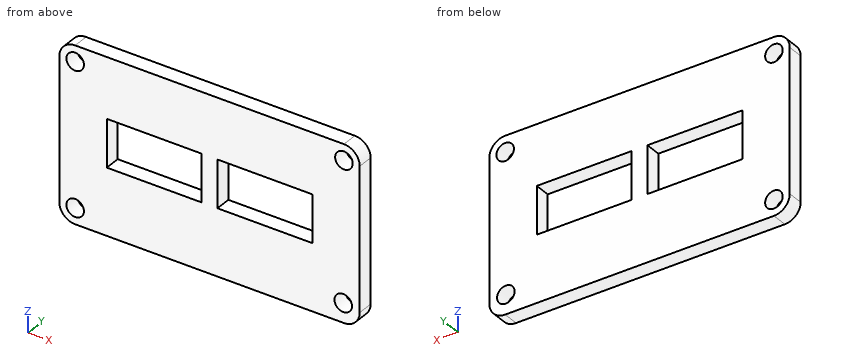
```python
from build123d import *

# Parameters (mm, degrees)
SKETCH1_W                   = 48.26
SKETCH1_H                   = 27.94
BOSS_EXTRUDE1_DEPTH         = 2.54
SKETCH2_W                   = 15.24
SKETCH2_H                   = 7.62
CUT_EXTRUDE1_DEPTH          = 15.494
FILLET1_R                   = 2.54
F_34_0_111_DIAMETER_HOLE1_D = 2.8194


with BuildPart() as part:
    # Sketch1 → Boss-Extrude1 (new body)
    with BuildSketch(Plane(origin=(0, 0, 0), x_dir=(1, 0, 0), z_dir=(0, 1, 0))):
        Rectangle(SKETCH1_W, SKETCH1_H)
    extrude(amount=BOSS_EXTRUDE1_DEPTH)

    # Sketch2 → Cut-Extrude1 (cut)
    with BuildSketch(Plane(origin=(0, 2.54, 0), x_dir=(1, 0, 0), z_dir=(0, 1, 0))):
        with Locations((-8.89, -0.508)):
            Rectangle(SKETCH2_W, SKETCH2_H)
        with Locations((8.89, -0.508)):
            Rectangle(SKETCH2_W, SKETCH2_H)
    extrude(amount=-CUT_EXTRUDE1_DEPTH, mode=Mode.SUBTRACT)

    # Fillet1
    fillet1_edges = [part.edges().sort_by_distance(p)[0] for p in [
        (-24.13, 1.27, 13.97),
        (-24.13, 1.27, -13.97),
        (24.13, 1.27, -13.97),
        (24.13, 1.27, 13.97),
    ]]
    fillet(fillet1_edges, radius=FILLET1_R)

    # #34 (0.111) Diameter Hole1 (through all)
    with Locations(Plane(origin=(0, 2.54, 0), x_dir=(1, 0, 0), z_dir=(0, 1, 0))):
        with Locations((21.483576639, 10.878336476), (21.59, -11.43), (-21.59, -11.43), (-21.59, 11.43)):
            Hole(F_34_0_111_DIAMETER_HOLE1_D / 2)


solid = part.part
```
Check sheet for the modelled part. Datum: model origin and axes. Units: mm. Give positions to 0.01 mm unless a question says otherwise; leave off trailing zeros. Loops run counter-clockwise (first coordinate to the right, second up) from the corner with the lowest first, then second, coordinate; pieces in that order, holes last. Notation, with made-up numbers: (-0.75, 30.5) - (6.25, 30.5) arc R26 ccw to (6.25, 48.5) - close; hole circle Ø2 at (72.25, 77.25). An arc over 180 degrees is marked (long way). One line per question, with ' | ' between items. Start each with the question number.
1. Material ranges on line 1 along X through (y, z) = (1.05, 2); line 2 along Z through (x, y) = (-21.59, 1.7); line 3 along Z through (x, y) = (-2, 0.9), recorded low to high. Write a range as [from, to].
2. Cross-section at B-B, the plane x = -6.5. Enter the section's corners in (y, z).
3. Gauge pin test, flat end, axial feed: pin 1 Ø2.5 at (x, z) = (-21.59, -11.43) entering from -Y. Record the tip position at first contact, or that the pin passes through.
4. Cross-section at C-C, the plane y = 1.85. Enter the section's corners in (x, z).
5. Cross-section at A-A, the plane z = 2.5. Enter the section's corners in (x, y).
Check result:
1) line 1: x = [-24.13, -16.51], [-1.27, 1.27], [16.51, 24.13] | line 2: z = [-13.97, -12.84], [-10.02, 10.02], [12.84, 13.97] | line 3: z = [-13.97, -3.3], [4.32, 13.97]
2) outline: (0, -13.97) - (2.54, -13.97) - (2.54, -3.3) - (0, -3.3) - close; (0, 4.32) - (2.54, 4.32) - (2.54, 13.97) - (0, 13.97) - close
3) pin 1: passes through
4) outline: (-24.13, -11.43) arc R2.54 ccw to (-21.59, -13.97) - (21.59, -13.97) arc R2.54 ccw to (24.13, -11.43) - (24.13, 11.43) arc R2.54 ccw to (21.59, 13.97) - (-21.59, 13.97) arc R2.54 ccw to (-24.13, 11.43) - close; hole circle Ø2.82 at (-21.59, -11.43); hole circle Ø2.82 at (-21.59, 11.43); hole (-16.51, -3.3) - (-1.27, -3.3) - (-1.27, 4.32) - (-16.51, 4.32) - close; hole (1.27, -3.3) - (16.51, -3.3) - (16.51, 4.32) - (1.27, 4.32) - close; hole circle Ø2.82 at (21.48, -10.88); hole circle Ø2.82 at (21.59, 11.43)
5) outline: (-24.13, 0) - (-16.51, 0) - (-16.51, 2.54) - (-24.13, 2.54) - close; (-1.27, 0) - (1.27, 0) - (1.27, 2.54) - (-1.27, 2.54) - close; (16.51, 0) - (24.13, 0) - (24.13, 2.54) - (16.51, 2.54) - close
